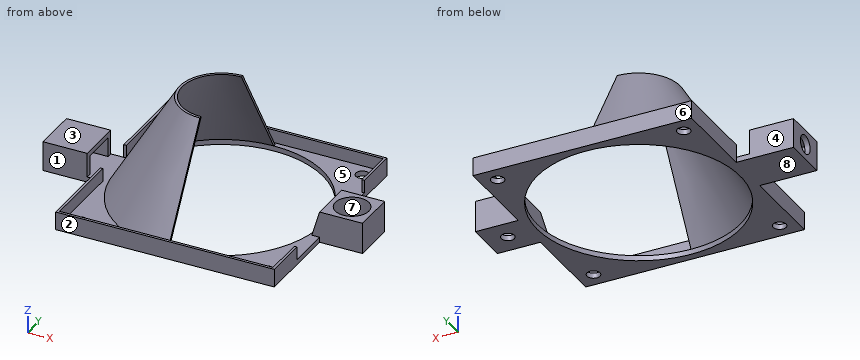
from build123d import *

# Parameters (mm, degrees)
CROQUIS1_W              = 84
CROQUIS1_H              = 84
CROQUIS1_R              = 39
CROQUIS1_R_2            = 2.5
SALIENTE_EXTRUIR1_DEPTH = 2
REVOLUCI_N2_ANGLE       = 180
SALIENTE_EXTRUIR2_DEPTH = 20
SALIENTE_EXTRUIR3_DEPTH = 15
CROQUIS8_W              = 11.4
CROQUIS8_H              = 17.5
CROQUIS8_R              = 3.6
SALIENTE_EXTRUIR4_DEPTH = 2
SALIENTE_EXTRUIR5_DEPTH = 16.5
CROQUIS10_W             = 16.5
CROQUIS10_H             = 16.5
CROQUIS10_R             = 6.45
SALIENTE_EXTRUIR6_DEPTH = 10
SALIENTE_EXTRUIR7_START = -16.5
SALIENTE_EXTRUIR7_DEPTH = 16.5
SALIENTE_EXTRUIR8_DEPTH = 5
CROQUIS13_R             = 2.5
CORTAR_EXTRUIR1_DEPTH   = 2


with BuildPart() as part:
    # Croquis1 → Saliente-Extruir1 (new body)
    with BuildSketch(Plane.XY):
        with Locations((-61.319838057, -7.506072874)):
            Rectangle(CROQUIS1_W, CROQUIS1_H)
        with Locations((-61.319838057, -7.506072874)):
            Circle(CROQUIS1_R, mode=Mode.SUBTRACT)
        with Locations((-97.028730507, 28.202819575)):
            Circle(CROQUIS1_R_2, mode=Mode.SUBTRACT)
        with Locations((-25.528730507, 28.202819575)):
            Circle(CROQUIS1_R_2, mode=Mode.SUBTRACT)
        with Locations((-25.528730507, -43.297180425)):
            Circle(CROQUIS1_R_2, mode=Mode.SUBTRACT)
        with Locations((-97.028730507, -43.297180425)):
            Circle(CROQUIS1_R_2, mode=Mode.SUBTRACT)
    extrude(amount=SALIENTE_EXTRUIR1_DEPTH)

    # Croquis4 → Revolución2 (revolve)
    with BuildSketch(Plane(origin=(-61.319838057, -49.506072874, 2), x_dir=(0, 0, -1), z_dir=(1, 0, 0))):
        Polygon((-40, 27), (0, 3), (0, 2), (-40, 26), align=None)
    revolve(axis=Axis((-61.319838057, -7.506072874, 2), (0, 0, -1)), revolution_arc=REVOLUCI_N2_ANGLE)

    # Croquis6 → Saliente-Extruir2 (add)
    with BuildSketch(Plane.ZY.offset(103.319838057)):
        Polygon((0, -7.506072874), (0, -16.256072874), (2, -16.256072874), (2, 1.243927126), (0, 1.243927126), align=None)
    extrude(amount=SALIENTE_EXTRUIR2_DEPTH)

    # Croquis7 → Saliente-Extruir3 (add)
    with BuildSketch(Plane.ZY.offset(123.319838057)):
        Polygon((11.4, 1.243927126), (2, 1.243927126), (2, -0.756072874), (9.4, -0.756072874), (9.4, -14.256072874), (2, -14.256072874), (2, -16.256072874), (11.4, -16.256072874), align=None)
    extrude(amount=-SALIENTE_EXTRUIR3_DEPTH)

    # Croquis8 → Saliente-Extruir4 (add)
    with BuildSketch(Plane.ZY.offset(123.319838057)):
        with Locations((5.7, -7.506072874)):
            Rectangle(CROQUIS8_W, CROQUIS8_H)
        with Locations((5.7, -7.506072874)):
            Circle(CROQUIS8_R, mode=Mode.SUBTRACT)
    extrude(amount=SALIENTE_EXTRUIR4_DEPTH)

    # Croquis9 → Saliente-Extruir5 (add)
    with BuildSketch(Plane(origin=(-19.319838057, 0, 0), x_dir=(0, 0, -1), z_dir=(1, 0, 0))):
        Polygon((0, -7.506072874), (0, 0.743927126), (-2, 0.743927126), (-2, -15.756072874), (0, -15.756072874), align=None)
    extrude(amount=SALIENTE_EXTRUIR5_DEPTH)

    # Croquis10 → Saliente-Extruir6 (add)
    with BuildSketch(Plane.XY.offset(2)):
        with Locations((-11.069838057, -7.506072874)):
            Rectangle(CROQUIS10_W, CROQUIS10_H)
        with Locations((-11.069838057, -7.506072874)):
            Circle(CROQUIS10_R, mode=Mode.SUBTRACT)
    extrude(amount=SALIENTE_EXTRUIR6_DEPTH)

    # Croquis11 → Saliente-Extruir7 (add)
    with BuildSketch(Plane(origin=(0, 0.743927126, 0), x_dir=(1, 0, 0), z_dir=(0, 1, 0)).offset(SALIENTE_EXTRUIR7_START)):
        Polygon((-19.319838057, -12), (-19.319838057, -2), (-22.319838057, -2), align=None)
    extrude(amount=SALIENTE_EXTRUIR7_DEPTH)

    # Croquis12 → Saliente-Extruir8 (add)
    with BuildSketch(Plane.XY.offset(2)):
        Polygon((-19.319838057, -32.631072874), (-20.319838057, -32.631072874), (-20.319838057, -48.506072874), (-102.319838057, -48.506072874), (-102.319838057, -16.256072874), (-103.319838057, -16.256072874), (-103.319838057, -49.506072874), (-19.319838057, -49.506072874), align=None)
        Polygon((-19.319838057, 34.493927126), (-103.319838057, 34.493927126), (-103.319838057, 1.243927126), (-102.319838057, 1.243927126), (-102.319838057, 33.493927126), (-20.319838057, 33.493927126), (-20.319838057, 17.618927126), (-19.319838057, 17.618927126), align=None)
    extrude(amount=SALIENTE_EXTRUIR8_DEPTH)

    # Croquis13 → Cortar-Extruir1 (cut)
    with BuildSketch(Plane.XY.offset(2)):
        with Locations((-11.069838057, -7.506072874)):
            Circle(CROQUIS13_R)
    extrude(amount=-CORTAR_EXTRUIR1_DEPTH, mode=Mode.SUBTRACT)


solid = part.part
Geometry check sheet. Reference: the model listing, model coordinates, mm. Face numbers are marked on the shaded views. A direction names the side the tool comes from. Round coordinates to 2 decimals unless told otherwise and drop trailing zeros. Order: outer loops, then holes, each group sorted by start corner. A loop starts at its lowest first (then second) coordinate and runs counter-clockwise, first axis right, second up. Notation, with made-up numbers: M 9.25,45.25 L 59.25,45.25 A12 cw 59.25,59.25 Z; hole C -24,43.5 d8. An arc over 180 degrees is marked long. Write each question's results on one line, items separated by ' | '. Start each with the question number.
1. Cross-section at A-A on x = -59. Record the boundary of the cut face in (y, z).
2. Draft check along Y on the marked faces 6, 7 and 8. Enter one of: pulls with the +Y half, pulls with the -Y half, needs draft (parallel to the pull), parting line crosses it, or undercut.
3. Cross-section at C-C on z = 21. Record the boundary of the cut face in (x, y), plus the area to 3 significant figures.
4. Set-up check for the marked faces 1, 2, 3, 4 and 5: record each of +Z, -Z, +X, -X, +Y, -Y from which the full face is reachable in a straight line by a thin tool's end or side.
5. Cross-section at D-D on z = 14. Record the boundary of the cut face in (x, y).
6. Go/stop test with flat-tipped pins: P1, Ø7.5, axis at y = 18.5, z = 3.5, coming from the +X side; P2, Ø3.5, axis at x = -114, z = 6, coming from the -Y side; P3, Ø12, axis at x = -111.5, y = 20.5, coming from the -Z side; P4, Ø5.5, axis at y = -40.5, z = 3.5, coming from the -X side. Record where each tip stops, or that it passes through.
7. Cross-section at B-B on z = 3.5. Give the number of separate pieces and of enclosed holes in the cut face, plus the area to 3 significant figures.
8. Material ranges on L1, parallel to Y at x = -34, z = 3; L2, parallel to Z at x = -102.5, y = 27; L3, parallel to Z at x = -90, y = -36.5, recorded low to high. Write a range as from..to.
Resolved:
1) outline: M -49.51,0 L -46.44,0 L -46.44,2 L -48.51,2 L -48.51,7 L -49.51,7 Z; M 31.42,0 L 34.49,0 L 34.49,7 L 33.49,7 L 33.49,2 L 31.42,2 Z
2) face 6: pulls with the +Y half | face 7: undercut | face 8: needs draft
3) outline: M -61.32,-36.11 L -61.32,-35.11 A27.6 cw -61.32,20.09 L -61.32,21.09 A28.6 ccw Z | area: 88.3 mm2
4) face 1: +Z, -Z, -X, -Y | face 2: +Z, -Z, +X, -X, -Y | face 3: +Z, -X, +Y, -Y | face 4: +Z, -Z, -X, +Y | face 5: none
5) outline: M -61.32,-40.31 L -61.32,-39.31 A31.8 cw -61.32,24.29 L -61.32,25.29 A32.8 ccw Z
6) P1: x = -19.32 | P2: y = -16.26 | P3: through | P4: x = -103.32
7) separate pieces: 6 | enclosed holes: 1 | area: 653 mm2
8) L1: -49.51..-48.51, 33.49..34.49 | L2: 0..7 | L3: 0..2
